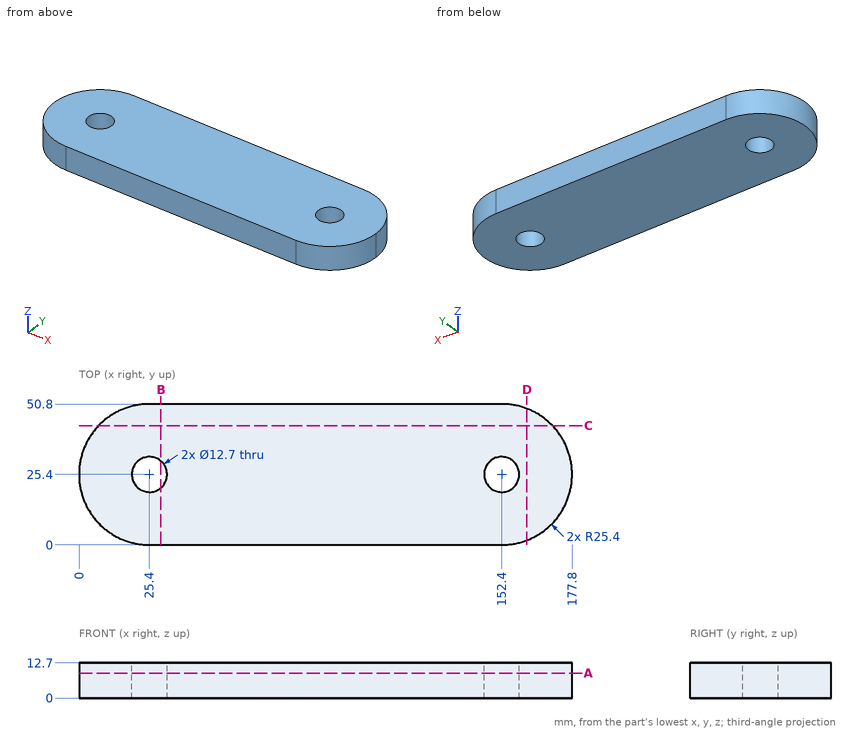
Job drawing, mm, ordinate dimensions from the low corner. One solid piece. Give positions to 0.01 mm unless a question says otherwise; leave off trailing zeros. Write each loop counter-clockwise with the first axis right and the second up, starting at its lowest first coordinate (ties: lowest second). Pieces come first, ordered by that corner, then holes. Notation, with made-up numbers: (38.5, 43.25) -> (80.5, 43.25) arc R20 ccw to (80.5, 72.25) -> close; hole circle Ø5 at (29, 52.5). An arc over 180 degrees is marked (long way). Return JSON: item names as keys, results as strings.
Item 1: Band-saw the part on C-C (y = 43). List the corners of the cut face in (x, z).
Answer below:
{"outline": "(7.09, 0) -> (170.71, 0) -> (170.71, 12.7) -> (7.09, 12.7) -> close"}
Item 2: Drop flat-ended pins along their axis: pin 1 (10 mm diameter, centred on x = 152.4, y = 25.4, fed in from +Z); pin 2 (2 mm diameter, centred on y = 35.5, z = 9, fed in from +X). Give the stop position or say it passes through.
Answer below:
{"pin 1": "passes through", "pin 2": "stops at x = 176.11"}
Item 3: Drill centre lines: probe 1 along Y at (x, z) = (152.4, 6); probe 2 along Y at (x, z) = (156.5, 9); probe 3 along X at (y, z) = (36, 8.25). Where is each one in solid material? Low to high.
Answer below:
{"probe 1": "y = 0 to 19.05, 31.75 to 50.8", "probe 2": "y = 0.33 to 20.55, 30.25 to 50.47", "probe 3": "x = 2.32 to 175.48"}
Item 4: Band-saw the part on D-D (x = 161.5). List the corners of the cut face in (y, z).
Answer below:
{"outline": "(1.69, 0) -> (49.11, 0) -> (49.11, 12.7) -> (1.69, 12.7) -> close"}
Item 5: Band-saw the part on A-A (z = 9). List the corners of the cut face in (x, y).
Answer below:
{"outline": "(25.4, 0) -> (152.4, 0) arc R25.4 ccw to (177.8, 25.4) arc R25.4 ccw to (152.4, 50.8) -> (25.4, 50.8) arc R25.4 ccw to start; hole circle Ø12.7 at (25.4, 25.4); hole circle Ø12.7 at (152.4, 25.4)"}
Item 6: Band-saw the part on B-B (x = 29.5). List the corners of the cut face in (y, z).
Answer below:
{"outline": "(0, 0) -> (20.55, 0) -> (20.55, 12.7) -> (0, 12.7) -> close; (30.25, 0) -> (50.8, 0) -> (50.8, 12.7) -> (30.25, 12.7) -> close"}
